Could you check a few things on this model? Use its own coordinates, in mm. Coordinates: 2 decimals unless noted, no trailing zeros. Write each loop counter-clockwise with the first axis right and the second up, starting at its lowest first coordinate (ties: lowest second). Pieces come first, ordered by that corner, then holes.
Item 1: I want a section at B-B on x = 3.5. Please give me the cut outline in (y, z), then the cut area to 3 significant figures.
Item 2: I want a section at C-C on z = 4.25. Please give me the cut outline in (x, y), then the cut area to 3 significant figures.
Item 3: For P1, Ø1.5, axis at x = 5, z = 2, coming from the +Y side, with a flat end and sliding along its axis, tell me the tip position at first contact or that it passes through.
Item 4: If I drill on probe 1 along Z at (x, y) = (-2.5, -0.1); probe 2 along X at (y, z) = (-0.2, 4.25); probe 3 along Z at (x, y) = (8.5, -0.55), over which ranges is the centre line in solid material (lowest first)?
from build123d import *

# Parameters (mm, degrees)
F1_DEPTH = 1


with BuildPart() as f1:
    # F0 (on Front) → F1 (new body)
    with BuildSketch(Plane.XZ):
        with BuildLine():
            Line((10, -15), (10, 0))
            ThreePointArc((10, 0), (0, 10), (-10, 0))
            Line((-10, 0), (-10, -15))
            Line((-10, -15), (10, -15))
        make_face()
        with BuildLine():
            ThreePointArc((9.684985, -2.490193), (9.680742, -2.506638), (9.676471, -2.523077))
            Line((9.676471, -2.523077), (9.676471, -2.490193))
            Line((9.676471, -2.490193), (9.684985, -2.490193))
        make_face(mode=Mode.SUBTRACT)
    extrude(amount=F1_DEPTH)


solid = f1.part
Response values:
1. outline: (-1, -15) - (0, -15) - (0, 9.37) - (-1, 9.37) - close
1. area: 24.4 mm2
2. outline: (-9.05, -1) - (9.05, -1) - (9.05, 0) - (-9.05, 0) - close
2. area: 18.1 mm2
3. P1: stops at y = 0
4. probe 1: z = -15 to 9.68
4. probe 2: x = -9.05 to 9.05
4. probe 3: z = -15 to 5.27
